For this review, take the finished solid that the model builds, in its own axes (mm). Round coordinates to 2 decimals unless told otherwise and drop trailing zeros. Order: outer loops, then holes, each group sorted by start corner. A loop starts at its lowest first (then second) coordinate and runs counter-clockwise, first axis right, second up. Notation, with made-up numbers: (51, 54.25) - (97, 54.25) arc R35 ccw to (97, 92.25) - close; hole circle Ø7 at (68.25, -38). An arc over 180 degrees is marked (long way). One line per item, written item: value.
Autodesk Fusion 360 part; units mm, degrees
sketch "Sketch1" plane through (0, 0, 0) normal (1, 0, 0) x (0, 1, 0)
  circle A0 centre (0, 0) radius 0.5
  line L0 (0.325, -0.325) -> (-0.325, -0.325)
  line L1 (-0.325, -0.325) -> (-0.325, 0.325)
  line L2 (-0.325, 0.325) -> (0.325, 0.325)
  line L3 (0.325, 0.325) -> (0.325, -0.325)
  line L4 (0.325, -0.325) -> (-0.325, 0.325) construction
  line L5 (-0.325, -0.325) -> (0.325, 0.325) construction
  dimension "d1" = 1
  dimension "d2" = 0.65
  dimension "d3" = 0.65
extrude "Extrude1" add sketch "Sketch1" along normal blind 38 contours A0 | L0 L1 L2 L3
sketch "Sketch2" plane through (38, 0, 0) normal (1, 0, 0) x (0, 1, 0)
  circle A0 centre (0, 0) radius 0.5
  line L0 (0.325, -0.325) -> (-0.325, -0.325)
  line L1 (-0.325, -0.325) -> (-0.325, 0.325)
  line L2 (-0.325, 0.325) -> (0.325, 0.325)
  line L3 (0.325, 0.325) -> (0.325, -0.325)
  line L4 (0.325, -0.325) -> (-0.325, 0.325) construction
  line L5 (-0.325, -0.325) -> (0.325, 0.325) construction
  dimension "d8" = 0.65
  dimension "d9" = 0.65
extrude "Extrude2" add sketch "Sketch2" along normal blind 1.645 contours L0 L1 L2 L3
extrude "Extrude3" add sketch "Sketch1" against normal blind 1.645 contours L0 L1 L2 L3
sketch "Sketch3" plane through (0, 0, -0.325) normal (0, 0, -1) x (1, 0, 0)
  line L0 (38, 0.325) -> (38, -0.325)
  line L1 (38, -0.325) -> (39.645, -0.325)
  line L2 (39.645, -0.325) -> (39.645, 0.325)
  line L3 (39.645, 0.325) -> (38, 0.325)
  line L4 (39.645, 0.325) -> (38.995, 0.325)
  line L5 (38.995, 0.325) -> (38.995, -0.325)
  line L6 (38.995, -0.325) -> (39.645, -0.325)
  line L7 (39.645, -0.325) -> (39.645, 0.325)
  line L8 (39.645, 0.325) -> (38.995, -0.325) construction
  line L9 (38.995, 0.325) -> (39.645, -0.325) construction
  point P0 (39.32, 0)
  dimension "d14" = 0.65
  dimension "d15" = 0.65
sketch "Sketch4" plane through (0, 0, -0.325) normal (0, 0, -1) x (1, 0, 0)
  line L0 (0, -0.325) -> (0, 0.325)
  line L1 (0, 0.325) -> (-1.645, 0.325)
  line L2 (-1.645, 0.325) -> (-1.645, -0.325)
  line L3 (-1.645, -0.325) -> (0, -0.325)
  line L4 (-0.995, -0.325) -> (-1.645, -0.325)
  line L5 (-1.645, -0.325) -> (-1.645, 0.325)
  line L6 (-1.645, 0.325) -> (-0.995, 0.325)
  line L7 (-0.995, 0.325) -> (-0.995, -0.325)
  line L8 (-0.995, -0.325) -> (-1.645, 0.325) construction
  line L9 (-1.645, -0.325) -> (-0.995, 0.325) construction
  point P0 (-1.32, 0)
  dimension "d17" = 0.65
  dimension "d18" = 0.65
extrude "Extrude4" add sketch "Sketch4" sketch "Sketch3" along normal blind 2.75 contours L1 L2 L3 L4 L5 L6 L7 of sketch 2 contours L1 L2 L3 L4 L5 L6 L7
fillet "Fillet1" radius 0.5 2 edges at (-0.995, 0, -0.325) (38.995, 0, -0.325)
fillet "Fillet2" radius 1 2 edges at (-1.645, 0, 0.325) (39.645, 0, 0.325)
fillet "Fillet3" radius 0.2 32 edges at (-1.32, -0.325, -3.075) (-0.995, 0, -3.075) (-1.32, 0.325, -3.075) (-1.645, 0, -3.075) (-0.8486, -0.325, -0.4714) (-0.995, -0.325, -1.95) (-0.2475, -0.325, -0.325) (-0.3225, -0.325, 0.325) (-1.3521, -0.325, 0.0321) (-1.645, -0.325, -1.875) (-0.3225, 0.325, 0.325) (-1.3521, 0.325, 0.0321) (-1.645, 0.325, -1.875) (-0.8486, 0.325, -0.4714) (-0.2475, 0.325, -0.325) (-0.995, 0.325, -1.95) (38.3225, -0.325, 0.325) (39.3521, -0.325, 0.0321) (39.645, -0.325, -1.875) (38.995, -0.325, -1.95) (38.8486, -0.325, -0.4714) (38.2475, -0.325, -0.325) (39.645, 0.325, -1.875) (39.3521, 0.325, 0.0321) (38.3225, 0.325, 0.325) (38.8486, 0.325, -0.4714) (38.995, 0.325, -1.95) (38.2475, 0.325, -0.325) (39.32, 0.325, -3.075) (39.645, 0, -3.075) (39.32, -0.325, -3.075) (38.995, 0, -3.075)
equation "d1 = width"
equation "d2 = d3"
equation "d3 = d1 * 0.65"
equation "width = 1 mm"
equation "baseLenght = 38 mm"
equation "d6 = baseLenght"
equation "d8 = width * 0.65"
equation "d9 = d8"
equation "d14 = width * 0.65"
equation "d15 = d14"
equation "d17 = width * 0.65"
equation "d18 = d17"
equation "d26 = 0.2 * width"
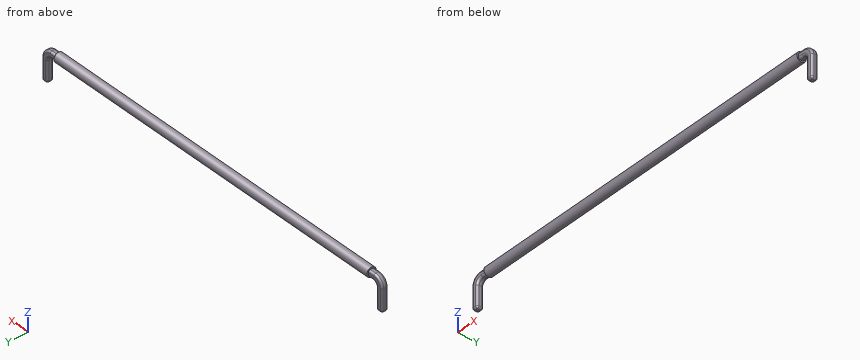
Item 1: For P1, Ø1.2, axis at x = -1, z = -2, coming from the -Y side (3 decimals); P2, Ø1, axis at x = 30.5, z = -1.5, coming from the -Y side, all flat-tipped, find the tip position at first contact; note any pin that passes through.
Returned:
P1: y = -0.325
P2: through
Item 2: Take a section at A-A (z = -2.3). Write out the cut boundary in (x, y) (3 decimals), plus the area to 3 significant figures.
Returned:
outline: (-1.645, -0.125) arc R0.2 ccw to (-1.445, -0.325) - (-1.195, -0.325) arc R0.2 ccw to (-0.995, -0.125) - (-0.995, 0.125) arc R0.2 ccw to (-1.195, 0.325) - (-1.445, 0.325) arc R0.2 ccw to (-1.645, 0.125) - close; (38.995, -0.125) arc R0.2 ccw to (39.195, -0.325) - (39.445, -0.325) arc R0.2 ccw to (39.645, -0.125) - (39.645, 0.125) arc R0.2 ccw to (39.445, 0.325) - (39.195, 0.325) arc R0.2 ccw to (38.995, 0.125) - close
area: 0.776 mm^2
Item 3: Wall thickness on line 1 (X direction, y = -0.05, z = -1.1) (3 decimals); line 2 (Z direction, x = 8, y = 0); line 3 (X direction, y = 0, z = -0.15): over which ranges is each line inside the solid? List them lowest first.
Returned:
line 1: -1.645 to -0.995, 38.995 to 39.645
line 2: -0.5 to 0.5
line 3: -1.5 to 39.5
Item 4: Take a section at B-B (x = 4). Write out the cut boundary in (y, z), plus the area to 3 significant figures.
Returned:
outline: circle Ø1 at (0, 0)
area: 0.785 mm^2
